Verification items for the finished model (mm, model axes). Face numbers are marked on the shaded views. A direction names the side the tool comes from. Coordinates: 2 decimals unless noted, no trailing zeros. Order: outer loops, then holes, each group sorted by start corner. A loop starts at its lowest first (then second) coordinate and runs counter-clockwise, first axis right, second up. Notation, with made-up numbers: (5.25, 83.25) -> (29.25, 83.25) arc R21 ccw to (29.25, 104.25) -> close; hole circle Ø3 at (32, 7.5). An arc over 180 degrees is marked (long way). Write each question's results on one line, items separated by ' | '. Start each with the question number.
(1) Cross-section at D-D on y = 3.5. Enter the section's corners in (x, z).
(2) Draft check along Y on the marked faces 1, 2 and 3. Enter one of: +Y half, -Y half, draft (parallel to the pull), parting line (faces both ways), or undercut.
(3) Cross-section at B-B on y = 1.75. Enter the section's corners in (x, z).
(4) Cross-section at A-A on z = 0. Enter the section's corners in (x, y), and give its area (3 significant figures).
(5) Cross-section at C-C on x = 6.5. Give the number of separate pieces and of enclosed holes in the cut face, and give its area (3 significant figures).
(6) Go/stop test with flat-tipped pins: pin 1 (5 mm diameter, centred on x = 3.5, z = -2.5, fed in from +Y); pin 2 (1.2 mm diameter, centred on x = 4, z = -4, fed in from -Y); pin 3 (2.5 mm diameter, centred on x = 3.5, z = -4.5, fed in from +Y). Record where each tip stops, or that it passes through.
(7) Set-up check for the marked faces 4, 5 and 6: record each of +Z, -Z, +X, -X, +Y, -Y from which the full face is reachable in a straight line by a thin tool's end or side.
(8) Thickness scan on probe 1 along X at (y, z) = (1, -4.5); probe 2 along Z at (x, y) = (3.5, -4.25); probe 3 along Y at (x, z) = (-1.15, 0). Record the ranges inside material, lowest first. Write a range as [from, to].
```python
from build123d import *
from build123d.topology import SkipClean

# Parameters (mm, degrees)
SKETCH1_R           = 5.5
BOSS_EXTRUDE1_DEPTH = 0.5
BOSS_EXTRUDE2_DEPTH = 6.5
CIRPATTERN1_COUNT   = 6
SKETCH3_R           = 5.5
SKETCH3_R_2         = 2
BOSS_EXTRUDE3_DEPTH = 0.25
SKETCH4_R           = 1.5
SKETCH4_R_2         = 0.75
BOSS_EXTRUDE4_DEPTH = 2.5


with BuildPart() as part:
    # Sketch1 → Boss-Extrude1 (new body)
    with BuildSketch(Plane(origin=(0, 0, 0), x_dir=(0, 0, -1), z_dir=(1, 0, 0))):
        Circle(SKETCH1_R)
    extrude(amount=BOSS_EXTRUDE1_DEPTH)

    # Sketch2 → Boss-Extrude2 (add)
    with BuildSketch(Plane(origin=(0.5, 0, 0), x_dir=(0, 0, -1), z_dir=(1, 0, 0))):
        with BuildLine():
            Line((-5.5, 0), (-3.02, 0))
            Line((-3.02, 0), (-3.02, 0.25))
            Line((-3.02, 0.25), (-5.344155686, 0.25))
            ThreePointArc((-5.344155686, 0.25), (-5.184805145, 1.319202641), (-4.813771652, 2.334545455))
            Line((-4.813771652, 2.334545455), (-4.948737213, 2.4))
            ThreePointArc((-4.948737213, 2.4), (-5.360412982, 1.231248417), (-5.5, 0))
        make_face()
    boss_extrude2 = extrude(amount=BOSS_EXTRUDE2_DEPTH)

    # CirPattern1: Boss-Extrude2 ×6 about axis
    with SkipClean():  # keep this step's faces unmerged: merging them makes the solid invalid here
        cirpattern1_axis = Axis((0, 0, 0), (1, 0, 0))
        for i in range(1, CIRPATTERN1_COUNT):
            add(boss_extrude2.rotate(cirpattern1_axis, i * 360 / CIRPATTERN1_COUNT))

    # Sketch3 → Boss-Extrude3 (add)
    with BuildSketch(Plane(origin=(7, 0, 0), x_dir=(0, 0, -1), z_dir=(1, 0, 0))):
        Circle(SKETCH3_R)
        Circle(SKETCH3_R_2, mode=Mode.SUBTRACT)
    extrude(amount=BOSS_EXTRUDE3_DEPTH)

    # Sketch4 → Boss-Extrude4 (add)
    with SkipClean():  # keep this step's faces unmerged: merging them makes the solid invalid here
        with BuildSketch(Plane.ZY):
            with Locations(Location((0, 0, 0), (0, 0, 180))):  # turned: the seam where the file's is
                Circle(SKETCH4_R)
            Circle(SKETCH4_R_2, mode=Mode.SUBTRACT)
        extrude(amount=BOSS_EXTRUDE4_DEPTH)


solid = part.part
```
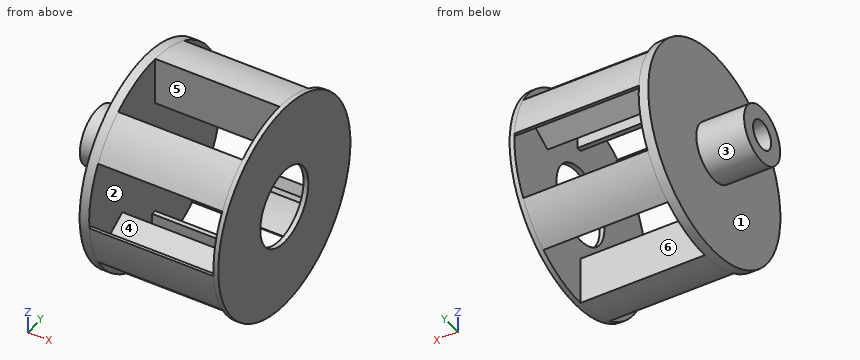
Results are:
1) outline: (0, -4.24) -> (7.25, -4.24) -> (7.25, 4.24) -> (7, 4.24) -> (7, 2.02) -> (0.5, 2.02) -> (0.5, 4.24) -> (0, 4.24) -> close; hole (0.5, -4.05) -> (7, -4.05) -> (7, -2.31) -> (0.5, -2.31) -> close; hole (0.5, -2.02) -> (7, -2.02) -> (7, 1.73) -> (0.5, 1.73) -> close
2) face 1: draft | face 2: undercut | face 3: parting line
3) outline: (0, -5.21) -> (0.5, -5.21) -> (0.5, 5.06) -> (7, 5.06) -> (7, 0.97) -> (7.25, 0.97) -> (7.25, 5.21) -> (0, 5.21) -> close; (7, -5.21) -> (7.25, -5.21) -> (7.25, -0.97) -> (7, -0.97) -> close
4) outline: (-2.5, -1.5) -> (0, -1.5) -> (0, -5.5) -> (0.5, -5.5) -> (0.5, 5.5) -> (0, 5.5) -> (0, 1.5) -> (-2.5, 1.5) -> (-2.5, 0.75) -> (0, 0.75) -> (0, -0.75) -> (-2.5, -0.75) -> close; (7, -5.5) -> (7.25, -5.5) -> (7.25, -2) -> (7, -2) -> close; (7, 2) -> (7.25, 2) -> (7.25, 5.5) -> (7, 5.5) -> close | area: 11.0 mm2
5) separate pieces: 6 | enclosed holes: 0 | area: 5.70 mm2
6) pin 1: stops at y = 4.76 | pin 2: stops at y = -0.25 | pin 3: stops at y = 4.44
7) face 4: none | face 5: +Z | face 6: -Z
8) probe 1: x = [0, 0.5], [7, 7.25] | probe 2: z = [-2.45, -2.17], [2.45, 2.74], [3.25, 3.49] | probe 3: y = [-1.5, -0.75], [0.75, 1.5]
